Source: CAD feature listing. Evaluate the final solid. Frame: model axes, mm. Give positions to 0.01 mm unless a question says otherwise; leave off trailing zeros. Loops run counter-clockwise (first coordinate to the right, second up) from the corner with the lowest first, then second, coordinate; pieces in that order, holes last. Notation, with made-up numbers: (-10.5, 75) -> (38.5, 75) arc R26 cw to (38.5, 112) -> close; hole circle Ø10 at (62, 21). An arc over 180 degrees is marked (long way). Put each result on its own line as item: value.
Autodesk Inventor part; units mm, degrees
ref_plane "Work Plane1" through (0, 46, 0) normal (0, 1, 0) x (-1, 0, 0)
ref_plane "Work Plane2" through (31, 0, 0) normal (1, 0, 0) x (0, 1, 0)
ref_plane "Work Plane3" through (31, 20, -31) normal (-0.9449861, -0.3271106, 0) x (0.3271106, -0.9449861, 0)
sketch "Sketch1" plane through (0, 0, 0) normal (0, 1, 0) x (-1, 0, 0)
  circle A0 centre (0, 0) radius 31
  dimension "d0" = 62
extrude "Extrusion1" add sketch "Sketch1" along normal blind 20
sketch "Sketch2" plane through (0, 20, 0) normal (0, 1, 0) x (1, 0, 0)
  line L0 (0, 0) -> (31.1009, 0)
  circle A0 centre (0, 0) radius 31
ref_plane "Work Plane1" through (0, 46, 0) normal (0, 1, 0) x (-1, 0, 0)
ref_plane "Work Plane2" through (31, 0, 0) normal (1, 0, 0) x (0, 1, 0)
sketch "Sketch3" plane through (0, 46, 0) normal (0, 1, 0) x (-1, 0, 0)
  circle A0 centre (0, 0) radius 31 construction
  line L0 (0, 0) -> (-22, 0)
  circle A1 centre (0, 0) radius 22
  dimension "d5" = 22
loft "Loft1" add profiles "Sketch3" section 1 edges at (31, 20, 0)
fillet "Fillet1" radius 8 1 edges at (22, 46, 0)
sketch "Sketch5" plane through (31, 0, 0) normal (1, 0, 0) x (0, 1, 0)
  line L0 (40.6169, -23.8634) -> (40.6169, 23.8634)
  line L1 (20, -31) -> (20, 31)
  point P0 (0, 0)
ref_plane "Work Plane3" through (31, 20, -31) normal (-0.9449861, -0.3271106, 0) x (0.3271106, -0.9449861, 0)
sketch "Sketch6" plane through (31, 20, -31) normal (-0.9449861, -0.3271106, 0) x (0.3271106, -0.9449861, 0)
  ellipse E0 centre (-29.6231, 31) end of major axis (-29.6231, 54.8634) minor radius 7.806 construction
  line L0 (34.5454, 31) -> (-68.4133, 31) construction
  point P0 (8.7593, 31)
  point P1 (-11.8171, 31)
  point P2 (-21.8171, 31)
  dimension "d11" = 10
hole "Hole1" at (27.1345, 31.167, 0) direction (-0.9449861, -0.3271106, 0) diameter 9 depth 10 tip angle 118
thread "Thread1"
sketch "Sketch7" plane through (0, 46, 0) normal (0, 1, 0) x (1, 0, 0)
  circle A0 centre (0, 0) radius 12.5
  dimension "d21" = 25
sketch "Sketch8" plane through (0, 0, 0) normal (0, -1, 0) x (1, 0, 0)
  circle A0 centre (0, 0) radius 12.5
  dimension "d22" = 25
hole "Hole2" at (0, 0, 0) direction (0, 1, 0) diameter 25 end through all countersink diameter 28 countersink angle 45.49
thread "Thread2"
properties part number "ClampingNut" material "Polycarbonate, Clear"
(1) First-contact query: P1, Ø2, axis at x = -1, y = 23.5, coming from the -Z side; P2, Ø2, axis at x = 6, y = 33, coming from the -Z side; P3, Ø20, axis at x = 0, z = 0, coming from the -Y side; P4, Ø1, axis at x = 1, y = 39, coming from the +Z side. Flat tips, straight axial feed; report the tip coordinate or a pass-through.
Calculated:
P1: stops at z = -30.12
P2: stops at z = -26.23
P3: passes through
P4: stops at z = 24.58
(2) Draft query along Z for faces 1 (the conical face through (-12.294, 3.354, 2.73)), 2 (the cylindrical face through (4.036, 9.86, -30.736)), 3 (the conical face through (15.5, 27.39, -0.75)), 4 (the flat face through (-6, 0, -13)). Return one class per face: released by +Z, released by -Z, zero draft, split by the parting line, or undercut.
Calculated:
face 1: undercut
face 2: split by the parting line
face 3: undercut
face 4: zero draft
(3) Line query: probe 1 along Z at (x, y) = (0, 15.5); probe 2 along Z at (x, y) = (0, 26). Output: solid intervals per line, ascending. Write a range as from..to.
Calculated:
probe 1: z = -31..-12.5, 12.5..31
probe 2: z = -28.92..-12.5, 12.5..28.92
(4) Section B-B on y = 18.5. Return loops of the section in (x, z).
Calculated:
outline: circle Ø62 at (0, 0); hole circle Ø25 at (0, 0)
(5) Section A-A on x = 0. Return loops of the section in (y, z), then the cut area to 3 significant figures.
Calculated:
outline: (0, -31) -> (20, -31) -> (40.62, -23.86) arc R8 ccw to (46, -16.3) -> (46, -12.5) -> (3.58, -12.5) -> (0, -14) -> close; (0, 14) -> (3.58, 12.5) -> (46, 12.5) -> (46, 16.3) arc R8 ccw to (40.62, 23.86) -> (20, 31) -> (0, 31) -> close
area: 1,450 mm²
